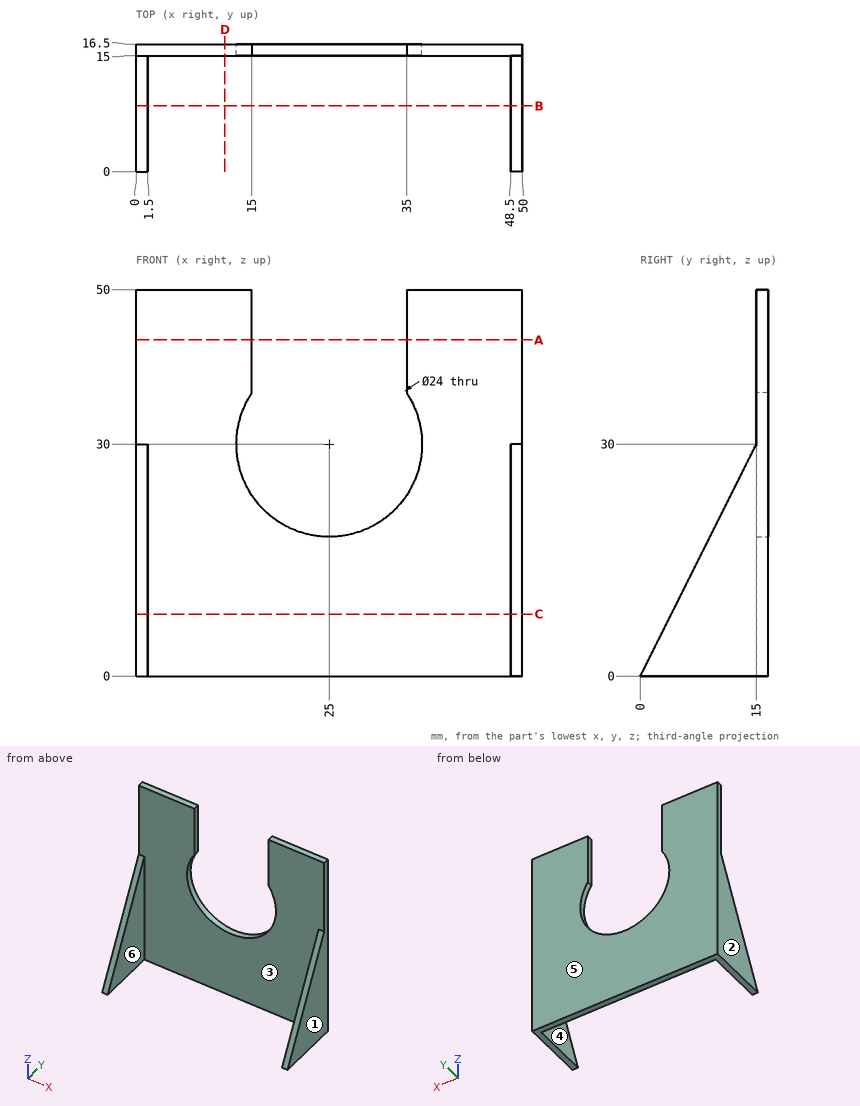
Source: three-view drawing plus pictorial views. Frame: mm from the lowest corner of the part. A direction names the side the tool comes from. Coordinates: 2 decimals unless noted, no trailing zeros. Loops run counter-clockwise (first coordinate to the right, second up) from the corner with the lowest first, then second, coordinate; pieces in that order, holes last. Notation, with made-up numbers: (22, 36) -> (55, 36) arc R25 cw to (55, 55) -> close; hole circle Ø2 at (38, 20.5). An arc over 180 degrees is marked (long way). Write each question's results on one line, items separated by ' | '. Start each with the question number.
Q1. Section D-D, the plane x = 11.5. Return the cut outline in (y, z), plus the area to 3 significant figures.
Q2. Section B-B, the plane y = 8.5. Return the cut outline in (x, z).
Q3. Reachability of the marked faces 5 and 6 from +Z, -Z, +X, -X, +Y, -Y: full face, straight path, thin tool, end or side. Return the list, or none.
Q4. Ray query, line 1 (X direction, y = 12.25, z = 8.5); line 2 (X direction, y = 15.35, z = 30); line 3 (Y direction, x = 5.5, z = 30.5). Return the intervals inside material, ascending. Write a range as from..to.
Q5. Pin query (flat end, axial travel): pin 1 (25 mm diameter, centred on x = 19.5, z = 24.5, fed in from -Y). Return the tip coordinate at first contact, or that it passes through.
Q6. Pull-direction query (X, two-part tool) for the marked faces 1, 2, 3 and 4; classes: released by +X, released by -X, zero draft, split by the parting line, or undercut.
Q7. Section C-C, the plane z = 8. Return the cut outline in (x, y), plus the area to 3 significant figures.
Q8. Section A-A, the plane z = 43.5. Return the cut outline in (x, y).
Found:
1) outline: (15, 0) -> (16.5, 0) -> (16.5, 50) -> (15, 50) -> close | area: 75.0 mm2
2) outline: (0, 0) -> (1.5, 0) -> (1.5, 17) -> (0, 17) -> close; (48.5, 0) -> (50, 0) -> (50, 17) -> (48.5, 17) -> close
3) face 5: +Z, -Z, +X, -X, +Y | face 6: +Z, -Z, -Y
4) line 1: 0..1.5, 48.5..50 | line 2: 0..13, 37..50 | line 3: 15..16.5
5) pin 1: y = 15
6) face 1: released by +X | face 2: released by -X | face 3: undercut | face 4: undercut
7) outline: (0, 4) -> (1.5, 4) -> (1.5, 15) -> (48.5, 15) -> (48.5, 4) -> (50, 4) -> (50, 16.5) -> (0, 16.5) -> close | area: 108 mm2
8) outline: (0, 15) -> (15, 15) -> (15, 16.5) -> (0, 16.5) -> close; (35, 15) -> (50, 15) -> (50, 16.5) -> (35, 16.5) -> close
